Could you check a few things on this model? Use its own coordinates, in mm. Face numbers are marked on the shaded views. Round coordinates to 2 decimals unless told otherwise and drop trailing zeros. Loops run counter-clockwise (first coordinate to the right, second up) from the corner with the lowest first, then second, coordinate; pieces in that order, holes last. Notation, with made-up numbers: (84, -40) -> (98, -40) arc R20 cw to (98, -18) -> close; hole circle Ø1 at (87.5, 64). An arc over 180 degrees is marked (long way). Write each question's results on one line, items separated by ' | '. Start each with the question number.
1) For P1, Ø4, axis at x = -31.75, y = 64.63, coming from the -Z side; P2, Ø3, axis at x = -36, y = 6, coming from the -Z side; P3, Ø4, axis at y = 42, z = 3, coming from the -X side; P4, Ø5, axis at y = -20, z = 1.5, coming from the -X side, each with a flat end and sliding along its axis, tell me the tip position at first contact or that it passes through.
2) Imagine slicing it at C-C, the plane z = 9. List the corners of the cut face in (x, y) for me, plus the area to 3 significant figures.
3) Imagine slicing it at D-D, the plane x = -21.5. List the corners of the cut face in (y, z) for me, plus the area to 3 significant figures.
4) We'd pull the mould along Y, two halves only. Please class the marked faces 1, 2, 3 and 4: pulls with the +Y half, pulls with the -Y half, needs draft (parallel to the pull), parting line crosses it, or undercut.
5) Imagine slicing it at A-A, the plane y = -23.5. List the corners of the cut face in (x, z) for me.
6) Imagine slicing it at B-B, the plane x = -10.5. List the corners of the cut face in (y, z) for me.
7) If I drill on probe 1 along X at (y, z) = (33, 2); probe 2 along X at (y, z) = (52, 3.25); probe 3 along X at (y, z) = (-22.5, 3.75), over which ranges is the centre line in solid material (lowest first)?
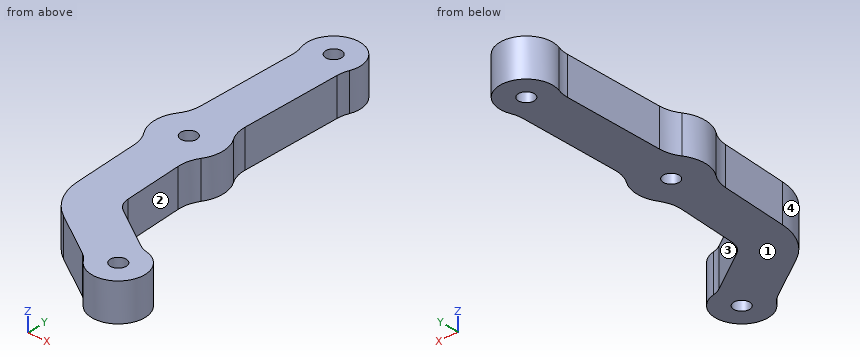
from build123d import *

# Parameters (mm, degrees)
CROQUIS1_R              = 2.1
SALIENTE_EXTRUIR1_DEPTH = 10


with BuildPart() as part:
    # Croquis1 → Saliente-Extruir1 (new body)
    with BuildSketch(Plane.XY):
        with BuildLine():
            Line((-38.297463257, 12.43995528), (-37.260227552, -5.729430968))
            ThreePointArc((-37.260227552, -5.729430968), (-35.302123155, -12.327326048), (-30.603607028, -17.356276091))
            Line((-30.603607028, -17.356276091), (-18.21840671, -25.610918133))
            ThreePointArc((-18.21840671, -25.610918133), (-17.187574321, -26.449545076), (-16.333802614, -27.467869404))
            ThreePointArc((-16.333802614, -27.467869404), (-4.742179488, -27.382198605), (-9.124005181, -16.65034556))
            ThreePointArc((-9.124005181, -16.65034556), (-10.39246616, -16.254217865), (-11.563209017, -15.625511598))
            Line((-11.563209017, -15.625511598), (-23.117754007, -7.92449503))
            ThreePointArc((-23.117754007, -7.92449503), (-24.683926049, -6.248178349), (-25.336627514, -4.048879989))
            Line((-25.336627514, -4.048879989), (-26.253353052, 12.009514726))
            ThreePointArc((-26.253353052, 12.009514726), (-25.979466195, 14.783004808), (-24.870216746, 17.339726714))
            ThreePointArc((-24.870216746, 17.339726714), (-23.472468719, 22.17483806), (-24.889381967, 27.004367864))
            ThreePointArc((-24.889381967, 27.004367864), (-25.965866103, 29.399778244), (-26.305025758, 32.003963281))
            Line((-26.305025758, 32.003963281), (-25.84900792, 58.962467928))
            ThreePointArc((-25.84900792, 58.962467928), (-25.680378416, 60.550833412), (-25.233618645, 62.084373932))
            ThreePointArc((-25.233618645, 62.084373932), (-31.635589461, 71.629913394), (-38.356741428, 62.306358804))
            ThreePointArc((-38.356741428, 62.306358804), (-37.962103741, 60.758585549), (-37.847291474, 59.165425451))
            Line((-37.847291474, 59.165425451), (-38.303309312, 32.206920805))
            ThreePointArc((-38.303309312, 32.206920805), (-38.73035213, 29.615696581), (-39.887236501, 27.25806491))
            ThreePointArc((-39.887236501, 27.25806491), (-41.472447055, 22.148538835), (-39.877642432, 17.041999163))
            ThreePointArc((-39.877642432, 17.041999163), (-38.770646544, 14.849791642), (-38.297463257, 12.43995528))
        make_face()
        with Locations((-10.567, -23.5)):
            Circle(CROQUIS1_R, mode=Mode.SUBTRACT)
        with Locations((-32.472451023, 22.156990874)):
            Circle(CROQUIS1_R, mode=Mode.SUBTRACT)
        with Locations((-31.753981392, 64.630914655)):
            Circle(CROQUIS1_R, mode=Mode.SUBTRACT)
    extrude(amount=SALIENTE_EXTRUIR1_DEPTH)


solid = part.part
Checked values:
1) P1: through | P2: z = 0 | P3: x = -38.17 | P4: x = -30.39
2) outline: (-39.89, 27.26) arc R9 ccw to (-39.88, 17.04) arc R9 cw to (-38.3, 12.44) -> (-37.26, -5.73) arc R15 ccw to (-30.6, -17.36) -> (-18.22, -25.61) arc R7 cw to (-16.33, -27.47) arc R7 ccw (long way) to (-9.12, -16.65) arc R7 cw to (-11.56, -15.63) -> (-23.12, -7.92) arc R5 cw to (-25.34, -4.05) -> (-26.25, 12.01) arc R9 cw to (-24.87, 17.34) arc R9 ccw to (-24.89, 27) arc R9 cw to (-26.31, 32) -> (-25.85, 58.96) arc R9 cw to (-25.23, 62.08) arc R7 ccw (long way) to (-38.36, 62.31) arc R9 cw to (-37.85, 59.17) -> (-38.3, 32.21) arc R9 cw to start; hole circle Ø4.2 at (-32.47, 22.16); hole circle Ø4.2 at (-31.75, 64.63); hole circle Ø4.2 at (-10.57, -23.5) | area: 1,360 mm^2
3) outline: (-23.42, 0) -> (-9, 0) -> (-9, 10) -> (-23.42, 10) -> close | area: 144 mm^2
4) face 1: needs draft | face 2: undercut | face 3: pulls with the +Y half | face 4: pulls with the -Y half
5) outline: (-21.39, 0) -> (-12.67, 0) -> (-12.67, 10) -> (-21.39, 10) -> close; (-8.47, 0) -> (-3.57, 0) -> (-3.57, 10) -> (-8.47, 10) -> close
6) outline: (-30.5, 0) -> (-25.6, 0) -> (-25.6, 10) -> (-30.5, 10) -> close; (-21.4, 0) -> (-16.21, 0) -> (-16.21, 10) -> (-21.4, 10) -> close
7) probe 1: -38.29 to -26.29 | probe 2: -37.97 to -25.97 | probe 3: -22.89 to -12.41, -8.72 to -3.64
